Verification items for the finished model (mm, model axes). Round coordinates to 2 decimals unless told otherwise and drop trailing zeros. Order: outer loops, then holes, each group sorted by start corner. A loop starts at its lowest first (then second) coordinate and runs counter-clockwise, first axis right, second up. Notation, with made-up numbers: M 82.5,52.5 L 101.5,52.5 A20 cw 101.5,59.5 Z; hole C 83.5,53 d1. An arc over 180 degrees is marked long. Use one line per item in the form item = value. Start each with the question number.
Item 1: Cross-section at A-A on y = 514. Enter the section's corners in (x, z).
Item 2: Release check for a two-part mould opening along X. For faces 1 (the flat face through (-29, 568.25, 68)), 2 (the cylindrical face through (74.19, 534.6, 16.48)), 3 (the cylindrical face through (64.76, 533.65, -33.69)) record: +X half, -X half, draft (parallel to the pull), parting line (faces both ways), or undercut.
Item 3: Go/stop test with flat-tipped pins: pin 1 Ø8 at (x, y) = (-39, 342.5) entering from +Z; pin 2 Ø4 at (y, z) = (504, -54.5) entering from -X; pin 3 Ø1.5 at (y, z) = (336, -52.5) entering from -X. Record where each tip stops, or that it passes through.
Item 4: Thickness scan on probe 1 along X at (y, z) = (521, 0); probe 2 along X at (y, z) = (399.5, 43); probe 3 along Z at (x, y) = (-12.5, 534) (3 decimals). Record the ranges inside material, lowest first. Write a range as [from, to].
from build123d import *

# Parameters (mm, degrees)
SKETCH4_R          = 2
CUT_EXTRUDE1_DEPTH = 598.137418243
SKETCH5_R          = 2
CUT_EXTRUDE2_DEPTH = 597.095224503
SKETCH6_R          = 2
CUT_EXTRUDE3_DEPTH = 597.095224503


with BuildPart() as part:
    # Sketch1 → Revolve2 (revolve)
    with BuildSketch(Plane.XY, mode=Mode.PRIVATE) as revolve2_sk:
        with BuildLine():
            Line((57.272319057, 300.990034), (60.272319057, 300.990034))
            add(Edge.make_bspline(
                [(60.272319057, 300.990034), (60.786580015, 305.295203792), (62.216459446, 317.463391064), (64.020877786, 333.572779096), (66.11894295, 353.631593101), (68.030132581, 373.329466343), (69.466784443, 389.09643856), (70.806129018, 404.87199461), (71.886996993, 418.683052253), (72.742662769, 430.526418849), (73.404435972, 440.399441684), (73.901071328, 448.299980017), (74.304775576, 455.214817724), (74.62677953, 461.143160456), (74.877801518, 466.084350078), (75.067577987, 470.037846817), (75.336303636, 476.005510657), (75.563352259, 481.736537174), (75.748085722, 487.230769759), (75.884662604, 492.488061525), (75.940348523, 495.116996281), (75.978043797, 497.370577281), (75.993594118, 498.87307617), (76, 499.624354134), (76, 500)],
                knots=[0.606633708, 0.606633708, 0.606633708, 0.606633708, 0.606633708, 0.640794795, 0.703164955, 0.734350023, 0.765535092, 0.796720055, 0.827905019, 0.859090157, 0.874682727, 0.890275296, 0.905867787, 0.921460278, 0.929256523, 0.937052769, 0.944849014, 0.95264526, 0.97632263, 0.982241972, 0.988161315, 0.994080657, 0.997040329, 1, 1, 1, 1, 1], degree=4))
            Line((76, 500), (76, 568.250034))
            Line((76, 568.250034), (73, 568.250034))
            Line((73, 568.250034), (73, 500))
            add(Edge.make_bspline(
                [(73, 500), (73, 499.624354134), (72.993594118, 498.87307617), (72.978043797, 497.370577281), (72.940348523, 495.116996281), (72.884662604, 492.488061525), (72.748085722, 487.230769759), (72.563352259, 481.736537174), (72.336303636, 476.005510657), (72.067577987, 470.037846817), (71.877801518, 466.084350078), (71.62677953, 461.143160456), (71.304775576, 455.214817724), (70.901071328, 448.299980017), (70.404435972, 440.399441684), (69.742662769, 430.526418849), (68.886996993, 418.683052253), (67.806129018, 404.87199461), (66.466784443, 389.09643856), (65.030132581, 373.329466343), (63.11894295, 353.631593101), (61.020877786, 333.572779096), (59.216459446, 317.463391064), (57.786580015, 305.295203792), (57.272319057, 300.990034)],
                knots=[0.636380793, 0.636380793, 0.636380793, 0.636380793, 0.636380793, 0.639340464, 0.642300135, 0.648219478, 0.654138821, 0.660058163, 0.683735533, 0.691531779, 0.699328024, 0.70712427, 0.714920515, 0.730513006, 0.746105497, 0.761698066, 0.777290636, 0.808475774, 0.839660738, 0.870845701, 0.90203077, 0.933215838, 0.995585998, 1.029747085, 1.029747085, 1.029747085, 1.029747085, 1.029747085], degree=4))
        make_face()
    revolve(revolve2_sk.sketch.rotate(Axis((0, 0, 0), (0, 1, 0)), 90), axis=Axis((0, 0, 0), (0, 1, 0)))

    # Sketch4 → Cut-Extrude1 (cut, through all)
    with BuildSketch(Plane(origin=(-53.74011537, 0, 53.74011537), x_dir=(0.7071067811865517, 0, 0.7071067811865435), z_dir=(-0.7071067811865435, 0, 0.7071067811865517))):
        with Locations((0, 564.250034)):
            Circle(SKETCH4_R)
    extrude(amount=-CUT_EXTRUDE1_DEPTH, mode=Mode.SUBTRACT)

    # Sketch5 → Cut-Extrude2 (cut, through all)
    with BuildSketch(Plane(origin=(-70.214844471, 0, -29.08394086), x_dir=(-0.3826834323650874, 0, 0.9238795325112878), z_dir=(-0.9238795325112878, 0, -0.3826834323650874))):
        with Locations((0, 564.250034)):
            Circle(SKETCH5_R)
    extrude(amount=-CUT_EXTRUDE2_DEPTH, mode=Mode.SUBTRACT)

    # Sketch6 → Cut-Extrude3 (cut, through all)
    with BuildSketch(Plane(origin=(-29.08394086, 0, -70.214844471), x_dir=(-0.9238795325112864, 0, 0.38268343236509067), z_dir=(-0.38268343236509067, 0, -0.9238795325112864))):
        with Locations((0, 564.250034)):
            Circle(SKETCH6_R)
    extrude(amount=-CUT_EXTRUDE3_DEPTH, mode=Mode.SUBTRACT)


solid = part.part
Output values:
q1.outline = C 0,0 d152; hole C 0,0 d146
q2.face_1 = draft
q2.face_2 = parting line
q2.face_3 = undercut
q3.pin_1 = 54.75
q3.pin_2 = -54.95
q3.pin_3 = -38.08
q4.probe_1 = [-76, -73], [73, 76]
q4.probe_2 = [-55.67, -51.82], [51.82, 55.67]
q4.probe_3 = [-74.965, -71.922], [71.922, 74.965]
